For this review, take the finished solid that the model builds, in its own axes (mm). Face numbers are marked on the shaded views. A direction names the side the tool comes from. Give positions to 0.01 mm unless a question says otherwise; leave off trailing zeros. Order: outer loops, then holes, each group sorted by start corner. A loop starts at its lowest first (then second) coordinate and runs counter-clockwise, first axis right, second up.
Item 1: Machinability: for the marked faces 5 and 6, which of the approach directions +Z, -Z, +X, -X, +Y, -Y give a long, thin tool a straight path to every point of the face, cutting with its end or side? Answer none if there is none.
Item 2: Consider section D-D (y = 5). Give the boundary of the cut face in (x, z), plus the area to 3 significant figures.
Item 3: Consider section A-A (y = 3). Give the boundary of the cut face in (x, z), plus the area to 3 significant figures.
Item 4: For probe 1 along Z at (x, y) = (13.5, 4.25); probe 2 along Y at (x, z) = (15, 1.35); probe 3 along X at (y, z) = (0.1, 7.5), list the stretches that pass through material, from the lowest coordinate up.
Item 5: Consider section C-C (x = 15). Give the boundary of the cut face in (y, z), plus the area to 3 significant figures.
Item 6: For P1, Ø1.5, axis at y = 8, z = 11, coming from the +X side; P2, Ø4.5, axis at x = 5.5, z = 6.5, coming from the +Y side; P3, Ø5.5, axis at y = 1.5, z = 7, coming from the +X side; P4, Ø1, axis at x = 1, z = 6.5, coming from the -Y side, all flat-tipped, find the tip position at first contact; note any pin that passes through.
Item 7: The part is to be moulded in two halves that separate along Z. For the marked faces 1, 2, 3 and 4, say which applies: released by +Z, released by -Z, zero draft, split by the parting line, or undercut.
```python
from build123d import *

# Parameters (mm, degrees)
CROQUIS1_R              = 1.6
SALIENTE_EXTRUIR1_DEPTH = 15
CROQUIS2_W              = 10
CROQUIS2_H              = 10
CORTAR_EXTRUIR1_DEPTH   = 20
REDONDEO1_R             = 5
CROQUIS3_R              = 1.974471168
CORTAR_EXTRUIR2_DEPTH   = 11.2
CROQUIS4_R              = 2.8
CORTAR_EXTRUIR3_DEPTH   = 3
CROQUIS6_W              = 8
CROQUIS6_H              = 15
CROQUIS6_R              = 1.974471168
SALIENTE_EXTRUIR2_DEPTH = 1


with BuildPart() as part:
    # Croquis1 → Saliente-Extruir1 (new body)
    with BuildSketch(Plane.XY):
        Polygon((0, 0), (10, 0), (10, -1), (20, -1), (20, 0), (20, 4), (20, 9), (10, 9), (10, 4), (0, 4), align=None)
        with Locations((15, 5)):
            Circle(CROQUIS1_R, mode=Mode.SUBTRACT)
    extrude(amount=SALIENTE_EXTRUIR1_DEPTH)

    # Croquis2 → Cortar-Extruir1 (cut)
    with BuildSketch(Plane(origin=(0, 9, 0), x_dir=(1, 0, 0), z_dir=(0, 1, 0))):
        with Locations((15, -7.5)):
            Rectangle(CROQUIS2_W, CROQUIS2_H)
    extrude(amount=-CORTAR_EXTRUIR1_DEPTH, mode=Mode.SUBTRACT)

    # Redondeo1
    redondeo1_edges = [part.edges().sort_by_distance(p)[0] for p in [
        (10, 4, 1.25),
        (10, 4, 13.75),
    ]]
    fillet(redondeo1_edges, radius=REDONDEO1_R - 0.0001)  # a hair under: the kernel refuses the full size

    # Croquis3 → Cortar-Extruir2 (cut)
    with BuildSketch(Plane(origin=(0, 4, 0), x_dir=(1, 0, 0), z_dir=(0, 1, 0))):
        with Locations(Location((5, -7.5, 0), (0, 0, 270))):
            Circle(CROQUIS3_R)
    extrude(amount=-CORTAR_EXTRUIR2_DEPTH, mode=Mode.SUBTRACT)

    # Croquis4 → Cortar-Extruir3 (cut)
    with BuildSketch(Plane(origin=(0, 4, 0), x_dir=(1, 0, 0), z_dir=(0, 1, 0))):
        with Locations(Location((5, -7.5, 0), (0, 0, 270))):
            Circle(CROQUIS4_R)
    extrude(amount=-CORTAR_EXTRUIR3_DEPTH, mode=Mode.SUBTRACT)

    # Croquis6 → Saliente-Extruir2 (add)
    with BuildSketch(Plane.XZ):
        with Locations((6, 7.5)):
            Rectangle(CROQUIS6_W, CROQUIS6_H)
        with Locations(Location((5, 7.5, 0), (0, 0, 90))):
            Circle(CROQUIS6_R, mode=Mode.SUBTRACT)
    extrude(amount=SALIENTE_EXTRUIR2_DEPTH)


solid = part.part
```
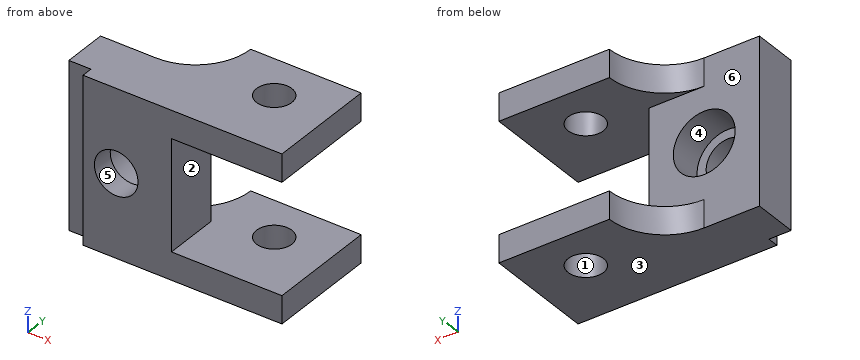
Resolved:
1. face 5: +Y, -Y
1. face 6: -X, +Y
2. outline: (8, 0) - (13.4, 0) - (13.4, 2.5) - (8, 2.5) - close; (8, 12.5) - (13.4, 12.5) - (13.4, 15) - (8, 15) - close; (16.6, 0) - (20, 0) - (20, 2.5) - (16.6, 2.5) - close; (16.6, 12.5) - (20, 12.5) - (20, 15) - (16.6, 15) - close
2. area: 44.0 mm2
3. outline: (0, 0) - (20, 0) - (20, 2.5) - (10, 2.5) - (10, 12.5) - (20, 12.5) - (20, 15) - (0, 15) - close; hole circle Ø5.6 at (5, 7.5)
3. area: 175 mm2
4. probe 1: z = 0 to 2.5, 12.5 to 15
4. probe 2: y = -1 to 3.4, 6.6 to 9
4. probe 3: x = 0 to 3.03, 6.97 to 10
5. outline: (-1, 0) - (3.4, 0) - (3.4, 2.5) - (-1, 2.5) - close; (-1, 12.5) - (3.4, 12.5) - (3.4, 15) - (-1, 15) - close; (6.6, 0) - (9, 0) - (9, 2.5) - (6.6, 2.5) - close; (6.6, 12.5) - (9, 12.5) - (9, 15) - (6.6, 15) - close
5. area: 34.0 mm2
6. P1: passes through
6. P2: stops at y = 4
6. P3: stops at x = 10
6. P4: stops at y = 0
7. face 1: zero draft
7. face 2: undercut
7. face 3: released by -Z
7. face 4: undercut
